Geometry check sheet. Reference: the model listing, model coordinates, mm. A direction names the side the tool comes from. Round coordinates to 2 decimals unless told otherwise and drop trailing zeros. Order: outer loops, then holes, each group sorted by start corner. A loop starts at its lowest first (then second) coordinate and runs counter-clockwise, first axis right, second up.
(1) Material ranges on line 1 along Y through (x, z) = (0.3, -1.35); line 2 along Z through (x, y) = (-1.15, 1.5); line 3 along Z through (x, y) = (-1.3, 1.25), recorded low to high.
(2) Go/stop test with flat-tipped pins: pin 1 (0.6 mm diameter, centred on x = -1.5, y = 1, fed in from +Z); pin 2 (1 mm diameter, centred on x = 1, z = 1, fed in from -Y); pin 3 (1.6 mm diameter, centred on y = 1, z = -2, fed in from +X); pin 4 (0.6 mm diameter, centred on x = -1, y = 1, fed in from -Z). Record where each tip stops, or that it passes through.
(3) Sectioned sample at A-A (x = 0). Record the boundary of the cut face in (y, z), plus the area to 3 significant figures.
(4) Sectioned sample at C-C (y = 7.25). Record the boundary of the cut face in (x, z).
(5) Set-up check for faces 1 (the face through (0.9, 0, 0.9)), 2 (the face through (0.5, 1, 1)), 3 (the face through (-1, 1, 0.5)): record each of +Z, -Z, +X, -X, +Y, -Y from which the full face is reachable in a straight line by a thin tool's end or side.
(6) Release check for a two-part mould opening along X. For faces 4 (the face through (-0.5, 1, 1)), 5 (the face through (-2.31, 7.41, 0.96)), 6 (the face through (0.5, 1, -1)), 7 (the face through (1, 1, 0.5)) record: +X half, -X half, draft (parallel to the pull), parting line (faces both ways), or undercut.
(7) Sectioned sample at B-B (z = 0). Record the boundary of the cut face in (x, y), plus the area to 3 significant figures.
Autodesk Inventor part; units mm, degrees
ref_plane "YZ Plane" through (0, 0, 0) normal (1, 0, 0) x (0, 1, 0)
ref_plane "XZ Plane" through (0, 0, 0) normal (0, 1, 0) x (-1, 0, 0)
ref_plane "XY Plane" through (0, 0, 0) normal (0, 0, 1) x (1, 0, 0)
sketch "Szkic1" plane through (0, 0, 0) normal (0, 1, 0) x (-1, 0, 0)
  circle A0 centre (0, 0) radius 4.25
  line L0 (1.1547, 2) -> (2.3094, 0)
  line L1 (2.3094, 0) -> (1.1547, -2)
  line L2 (1.1547, -2) -> (-1.1547, -2)
  line L3 (-1.1547, -2) -> (-2.3094, 0)
  line L4 (-2.3094, 0) -> (-1.1547, 2)
  line L5 (-1.1547, 2) -> (1.1547, 2)
  circle A1 centre (0, 0) radius 2.5
  dimension "d0" = 8.5
  dimension "d1" = 4
  dimension "d2" = 5
extrude "Wyciągnięcie proste4" add sketch "Szkic1" along normal blind 15 contours L0 L1 L2 L3 L4 L5 | A1
thread "Gwint2"
chamfer "Faza1" distance 1 angle 45 1 edges at (2.5, 15, 0)
chamfer "Faza2" distance 1 angle 45 1 edges at (2.5, 0, 0)
sketch "Szkic3" plane through (0, 0, 0) normal (0, -1, 0) x (1, 0, 0)
  circle A0 centre (0, 0) radius 2.5
  line L0 (2.5, 0) -> (-2.5, 0) construction
  line L1 (0, 2.5) -> (0, 0.5) construction
  line L2 (0.5, 2.5) -> (0.5, 2.4495) construction
  line L3 (-0.5, 2.5) -> (-0.5, 2.4495) construction
  line L4 (2.5, 0.5) -> (2.4495, 0.5) construction
  line L5 (2.5, -0.5) -> (2.4495, -0.5) construction
  circle A1 centre (0, 0) radius 2.5 construction
  line L6 (2.4495, 0.5) -> (0.5, 0.5)
  line L7 (2.4495, -0.5) -> (0.5, -0.5)
  line L8 (0.5, 2.4495) -> (0.5, 0.5)
  line L9 (-0.5, 2.4495) -> (-0.5, 0.5)
  line L10 (-0.5, 0.5) -> (-0.5, -0.5) construction
  line L11 (0.5, 0.5) -> (0.5, -0.5) construction
  line L12 (0.5, -0.5) -> (-0.5, -0.5) construction
  line L13 (-0.5, -0.5) -> (-0.5, -2.4495)
  line L14 (-2.4495, -0.5) -> (-2.5, -0.5) construction
  line L15 (-2.4495, 0.5) -> (-2.5, 0.5) construction
  line L16 (-0.5, -2.4495) -> (-0.5, -2.5) construction
  line L17 (0.5, -2.4495) -> (0.5, -2.5) construction
  line L18 (0.5, -0.5) -> (0.5, -2.4495)
  line L19 (0.5, 0.5) -> (-0.5, 0.5) construction
  line L20 (0, 0.5) -> (0, -2.5) construction
  line L21 (-0.5, -0.5) -> (-2.4495, -0.5)
  line L22 (-0.5, 0.5) -> (-2.4495, 0.5)
  dimension "d22" = 0.5
  dimension "d23" = 0.5
  dimension "d24" = 0.5
  dimension "d25" = 0.5
extrude "Wyciągnięcie proste5" cut sketch "Szkic3" against normal blind 2 contours A0 L7 L18 L13 L21 L22 L9 L8 L6
properties part number "M5x15" material "Aluminum 6061"
Answer below:
1. line 1: y = 2 to 15
1. line 2: z = -2.22 to -0.5, 0.5 to 2.22
1. line 3: z = -2.14 to -0.5, 0.5 to 2.14
2. pin 1: stops at z = 2.19
2. pin 2: stops at y = 0
2. pin 3: stops at x = 2.19
2. pin 4: stops at z = -2.4
3. outline: (2, -2.5) - (14, -2.5) - (15, -1.5) - (15, 1.5) - (14, 2.5) - (2, 2.5) - close
3. area: 64.0 mm2
4. outline: circle Ø5 at (0, 0)
5. face 1: +Z, -Z, +X, -X, -Y
5. face 2: +Z, -Z, -Y
5. face 3: +X, -X, -Y
6. face 4: undercut
6. face 5: parting line
6. face 6: undercut
6. face 7: draft
7. outline: (-2.5, 2) - (2.5, 2) - (2.5, 14) - (1.5, 15) - (-1.5, 15) - (-2.5, 14) - close
7. area: 64.0 mm2
